Source: CAD feature listing. Evaluate the final solid. Frame: model axes, mm. A direction names the side the tool comes from. Coordinates: 2 decimals unless noted, no trailing zeros. Order: outer loops, then holes, each group sorted by start corner. A loop starts at its lowest first (then second) coordinate and runs counter-clockwise, first axis right, second up.
```python
from build123d import *

# Parameters (mm, degrees)
SKETCH1_W                   = 355.6
SKETCH1_H                   = 101.6
EXTRUDE1_DEPTH              = 50.8
SKETCH6_W                   = 231.14
SKETCH6_H                   = 95.25
EXTRUDE2_DEPTH              = 12.7
FILLET1_R                   = 6.35
LPATTERN3_COUNT             = 2
LPATTERN3_PITCH             = 203.2
LPATTERN3_COUNT_DIR2        = 2
LPATTERN3_PITCH_DIR2        = 69.85
F_1_4_CLEARANCE_HOLE2_D     = 7.14248
F_1_4_CLEARANCE_HOLE2_DEPTH = 63.5
F_1_4_CLEARANCE_HOLE1_D     = 7.14248
LPATTERN4_COUNT             = 2
LPATTERN4_PITCH             = 50.8
LPATTERN4_COUNT_DIR2        = 2
LPATTERN4_PITCH_DIR2        = 304.8
CHAMFER1_SIZE               = 2.54


with BuildPart() as part:
    # Sketch1 → Extrude1 (new body)
    with BuildSketch(Plane.XY):
        Rectangle(SKETCH1_W, SKETCH1_H)
    extrude(amount=EXTRUDE1_DEPTH)

    # Sketch6 → Extrude2 (cut)
    with BuildSketch(Plane.XY.offset(50.8)):
        with Locations((1.27, 3.175)):
            Rectangle(SKETCH6_W, SKETCH6_H)
    extrude(amount=-EXTRUDE2_DEPTH, mode=Mode.SUBTRACT)

    # Fillet1
    fillet1_edges = [part.edges().sort_by_distance(p)[0] for p in [
        (116.84, -44.45, 44.45),
        (-114.3, -44.45, 44.45),
    ]]
    fillet(fillet1_edges, radius=FILLET1_R)

    # Sketch7 → 1/4-20 Tapped Hole1 (revolve, cut)
    with BuildSketch(Plane(origin=(101.6, -31.75, 38.1), x_dir=(0, -1, 0), z_dir=(1, 0, 0))):
        Polygon((0, 0), (0, 15.503816902), (2.5527, 13.97), (2.5527, 0.635), (3.1877, 0), align=None)
    f_1_4_20_tapped_hole1 = revolve(axis=Axis((101.6, -31.75, 44.45), (0, 0, -1)), mode=Mode.SUBTRACT)

    # LPattern3: 1_4-20 Tapped Hole1 2 × 2
    with Locations(*[(-i * LPATTERN3_PITCH, j * LPATTERN3_PITCH_DIR2, 0) for i in range(LPATTERN3_COUNT) for j in range(LPATTERN3_COUNT_DIR2) if (i, j) != (0, 0)]):
        add(f_1_4_20_tapped_hole1, mode=Mode.SUBTRACT)

    # 1/4 Clearance Hole2
    with Locations(Plane.ZY.offset(177.8)):
        with Locations((44.45, 3.175)):
            Hole(F_1_4_CLEARANCE_HOLE2_D / 2, depth=F_1_4_CLEARANCE_HOLE2_DEPTH)

    # 1/4 Clearance Hole1 (through all)
    with Locations(Plane.XZ.offset(50.8)):
        with Locations((0, 44.45)):
            Hole(F_1_4_CLEARANCE_HOLE1_D / 2)

    # Sketch14 → CBORE for 3/8 Socket Head Cap Screw1 (revolve, cut)
    with BuildSketch(Plane(origin=(152.4, 25.4, 0), x_dir=(0, 1, 0), z_dir=(1, 0, 0))):
        Polygon((0, 0), (0, 50.8), (5.0419, 50.8), (5.0419, 9.525), (7.9375, 9.525), (7.9375, 0.635), (8.5725, 0), align=None)
    cbore_for_3_8_socket_head_cap_screw1 = revolve(axis=Axis((152.4, 25.4, -6.35), (0, 0, 1)), mode=Mode.SUBTRACT)

    # LPattern4: CBORE for 3_8 Socket Head Cap Screw1 2 × 2
    with Locations(*[(-j * LPATTERN4_PITCH_DIR2, -i * LPATTERN4_PITCH, 0) for i in range(LPATTERN4_COUNT) for j in range(LPATTERN4_COUNT_DIR2) if (i, j) != (0, 0)]):
        add(cbore_for_3_8_socket_head_cap_screw1, mode=Mode.SUBTRACT)

    # Chamfer1
    chamfer1_edges = [part.edges().sort_by_distance(p)[0] for p in [
        (116.84, 50.8, 44.45),
        (-114.3, 50.8, 44.45),
        (177.8, -50.8, 25.4),
        (-177.8, -50.8, 25.4),
        (-177.8, 50.8, 25.4),
        (177.8, 50.8, 25.4),
    ]]
    chamfer(chamfer1_edges, length=CHAMFER1_SIZE)


solid = part.part
```
1. Section query C-C, the plane y = -25.4. Output: boundary loops of the cut face in (x, z) (1 decimal).
2. Material intervals for line 1 along X through (y, z) = (-25, 35); line 2 along Y through (x, z) = (-101, 29); line 3 along Y through (x, z) = (-152, 5), sorted ascending.
3. Section query A-A, the plane z = 44.45. Output: boundary loops of the cut face in (x, y).
4. Draft query along Y for faces 4 (the cylindrical face through (-154.784, -17.829, 5.018)), 5 (the flat face through (-2, -50.8, 25)), 6 (the flat face through (-2, 1, 0)), 7 (the flat face through (-147, 26, 9.525)). Return one class per face: +Y half, -Y half, draft (parallel to the pull), parting line (faces both ways), or undercut.
5. Section query B-B, the plane x = 0. Output: boundary loops of the cut face in (y, z), plus the area to 3 significant figures.
6. Section query D-D, the plane x = 43. Output: boundary loops of the cut face in (y, z), plus the area to 3 significant figures.
7. Access query for faces 1 (the cylindrical face through (147.4, 24.74, 29.87)), 2 (the cylindrical face through (144.53, 24.37, 5.02)), 3 (the cylindrical face through (-145.606, 4.248, 41.044)). Directions: +Z, -Z, +X, -X, +Y, -Y. A direction counts if a zero-diameter tool reaches every point of the face in a straight line with its end or side. Return the directions, or none.
8. Contact query for flat-ended pins moving along their axis: P1, Ø9.5, axis at x = 0, z = 44.45, coming from the +Y side; P2, Ø6, axis at x = -152.4, y = 25.4, coming from the -Z side (1 decimal); P3, Ø6.5, axis at x = -101.6, y = -31.75, coming from the -Z side; P4, Ø4, axis at x = -10.5, y = -5, coming from the +Z side. Output: stop coordinate, or through.
Answer key:
1. outline: (-177.8, 0) - (-161, 0) - (-160.3, 0.6) - (-160.3, 9.5) - (-157.4, 9.5) - (-157.4, 50.8) - (-177.8, 50.8) - close; (-147.4, 9.5) - (-144.5, 9.5) - (-144.5, 0.6) - (-143.8, 0) - (143.8, 0) - (144.5, 0.6) - (144.5, 9.5) - (147.4, 9.5) - (147.4, 50.8) - (116.8, 50.8) - (116.8, 38.1) - (-114.3, 38.1) - (-114.3, 50.8) - (-147.4, 50.8) - close; (157.4, 9.5) - (160.3, 9.5) - (160.3, 0.6) - (161, 0) - (177.8, 0) - (177.8, 50.8) - (157.4, 50.8) - close
2. line 1: x = -177.8 to -157.43, -147.37 to 147.37, 157.43 to 177.8
2. line 2: y = -50.8 to -34.23, -29.27 to 35.62, 40.58 to 50.8
2. line 3: y = -50.8 to -33.33, -17.47 to 17.47, 33.33 to 50.8
3. outline: (-177.8, -48.26) - (-175.26, -50.8) - (-3.57, -50.8) - (-3.57, -44.45) - (-107.95, -44.45) arc R6.35 cw to (-114.3, -38.1) - (-114.3, -0.4) - (-177.8, -0.4) - close; (-177.8, 6.75) - (-114.3, 6.75) - (-114.3, 48.26) - (-116.84, 50.8) - (-175.26, 50.8) - (-177.8, 48.26) - close; (3.57, -50.8) - (175.26, -50.8) - (177.8, -48.26) - (177.8, 48.26) - (175.26, 50.8) - (119.38, 50.8) - (116.84, 48.26) - (116.84, -38.1) arc R6.35 cw to (110.49, -44.45) - (3.57, -44.45) - close; hole circle Ø10.08 at (-152.4, -25.4); hole circle Ø10.08 at (-152.4, 25.4); hole circle Ø10.08 at (152.4, -25.4); hole circle Ø10.08 at (152.4, 25.4)
4. face 4: undercut
4. face 5: -Y half
4. face 6: draft
4. face 7: undercut
5. outline: (-50.8, 0) - (50.8, 0) - (50.8, 38.1) - (-44.45, 38.1) - (-44.45, 40.88) - (-50.8, 40.88) - close; (-50.8, 48.02) - (-44.45, 48.02) - (-44.45, 50.8) - (-50.8, 50.8) - close
5. area: 3,910 mm2
6. outline: (-50.8, 0) - (50.8, 0) - (50.8, 38.1) - (-44.45, 38.1) - (-44.45, 50.8) - (-50.8, 50.8) - close
6. area: 3,950 mm2
7. face 1: +Z, -Z
7. face 2: -Z
7. face 3: -X
8. P1: stops at y = -44.45
8. P2: passes through
8. P3: stops at z = 0
8. P4: stops at z = 38.1
